Build history of the part. All positions in model axes, mm. Face numbers are marked on the shaded views. Give positions to 0.01 mm unless a question says otherwise; leave off trailing zeros. Loops run counter-clockwise (first coordinate to the right, second up) from the corner with the lowest first, then second, coordinate; pieces in that order, holes last. Notation, with made-up numbers: M -39.5,-8.75 L -34.5,-8.75 A21 cw -34.5,10.25 Z; hole C 51,54 d4. An arc over 180 degrees is marked long. Answer in a Markdown table with one row per item. Add a question column.
```python
from build123d import *

# Parameters (mm, degrees)
BOSS_EXTRUDE1_DEPTH     = 2.5
CUT_EXTRUDE1_DEPTH      = 31.618621785
CUT_EXTRUDE1_DEPTH_BACK = 31.618621785
SKETCH3_W               = 44
SKETCH3_H               = 29
SKETCH3_R               = 1.125
CUT_EXTRUDE2_DEPTH      = 1
BOSS_EXTRUDE2_START     = 0.5
SKETCH3_5_R             = 1.125
BOSS_EXTRUDE2_DEPTH     = 0.5


with BuildPart() as part:
    # Sketch1 → Boss-Extrude1 (new body)
    with BuildSketch(Plane(origin=(0, 0, 0), x_dir=(1, 0, 0), z_dir=(0, 1, 0))):
        with BuildLine():
            Line((22, 17.5), (-22, 17.5))
            ThreePointArc((-22, 17.5), (-24.121320344, 16.621320344), (-25, 14.5))
            Line((-25, 14.5), (-25, 7.5))
            ThreePointArc((-25, 7.5), (-24.12566565, 0), (-25, -7.5))
            Line((-25, -7.5), (-25, -14.5))
            ThreePointArc((-25, -14.5), (-24.121320344, -16.621320344), (-22, -17.5))
            Line((-22, -17.5), (22, -17.5))
            ThreePointArc((22, -17.5), (24.121320344, -16.621320344), (25, -14.5))
            Line((25, -14.5), (25, -7.5))
            ThreePointArc((25, -7.5), (24.12566565, 0), (25, 7.5))
            Line((25, 7.5), (25, 14.5))
            ThreePointArc((25, 14.5), (24.121320344, 16.621320344), (22, 17.5))
        make_face()
    extrude(amount=-BOSS_EXTRUDE1_DEPTH)

    # Sketch2 → Cut-Extrude1 (cut, two sides: drawn at the far end of the back side and taken through both)
    with BuildSketch(Plane.XY.offset(-CUT_EXTRUDE1_DEPTH_BACK)):
        with BuildLine():
            Line((-25, -2.5), (25, -2.5))
            ThreePointArc((25, -2.5), (0, -2.25), (-25, -2.5))
        make_face()
    extrude(amount=CUT_EXTRUDE1_DEPTH + CUT_EXTRUDE1_DEPTH_BACK, mode=Mode.SUBTRACT)

    # Sketch3 → Cut-Extrude2 (cut)
    with BuildSketch(Plane(origin=(0, 0, 0), x_dir=(1, 0, 0), z_dir=(0, 1, 0))):
        Rectangle(SKETCH3_W, SKETCH3_H)
        with Locations(Location((-18.99479618, 11.49479618, 0), (0, 0, 270))):
            Circle(SKETCH3_R, mode=Mode.SUBTRACT)
        with Locations(Location((18.99479618, 11.49479618, 0), (0, 0, 270))):
            Circle(SKETCH3_R, mode=Mode.SUBTRACT)
        with Locations(Location((18.99479618, -11.49479618, 0), (0, 0, 270))):
            Circle(SKETCH3_R, mode=Mode.SUBTRACT)
        with Locations(Location((-18.99479618, -11.49479618, 0), (0, 0, 270))):
            Circle(SKETCH3_R, mode=Mode.SUBTRACT)
    extrude(amount=-CUT_EXTRUDE2_DEPTH, mode=Mode.SUBTRACT)

    # Sketch3_5 → Boss-Extrude2 (add)
    with BuildSketch(Plane(origin=(0, 0, 0), x_dir=(1, 0, 0), z_dir=(0, 1, 0)).offset(BOSS_EXTRUDE2_START)):
        with Locations(Location((-18.99479618, 11.49479618, 0), (0, 0, 270))):
            Circle(SKETCH3_5_R)
        with Locations(Location((18.99479618, 11.49479618, 0), (0, 0, 270))):
            Circle(SKETCH3_5_R)
        with Locations(Location((18.99479618, -11.49479618, 0), (0, 0, 270))):
            Circle(SKETCH3_5_R)
        with Locations(Location((-18.99479618, -11.49479618, 0), (0, 0, 270))):
            Circle(SKETCH3_5_R)
    extrude(amount=-BOSS_EXTRUDE2_DEPTH)


solid = part.part
```
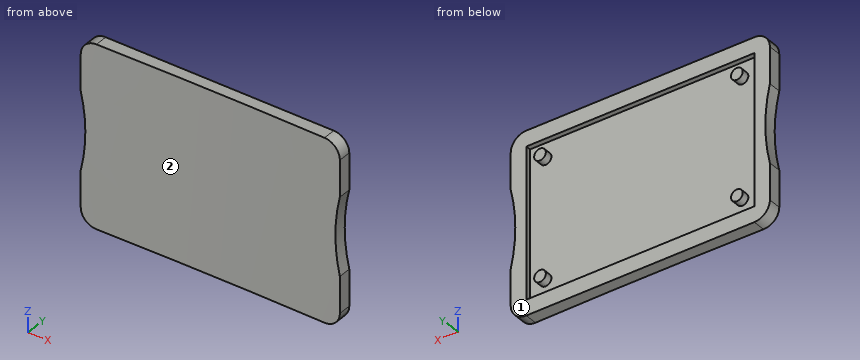
(1) Slice it at C-C, the plane z = -15. Give the cut face in (x, y) (3 decimals), then the cut area to 3 significant figures.
(2) Slice it at A-A, the plane x = -12.5. Give the cut face in (y, z).
(3) Pin check, flat tips, straight feed: pin 1 (0.5 mm diameter, centred on y = -0.5, z = 5, fed in from -X); pin 2 (2 mm diameter, centred on x = 1.5, z = 4, fed in from -Y); pin 3 (0.5 mm diameter, centred on y = -0.5, z = 2.5, fed in from +X). Stop position of each tip, or through.
(4) Wall check: line 1 (Z direction, x = -13, y = -0.5); line 2 (X direction, y = -0.1, z = 0); line 3 (Y direction, x = -2.5, z = 0.5). Give the ranges that are in metal, low to high.
(5) Pull direction X, two halves, no side cores. Call the marked faces 1 and 2: +X half, -X half, draft (parallel to the pull), parting line (faces both ways), or undercut.
(6) Slice it at B-B, the plane z = -8. Give the cut face in (x, y) (3 decimals), then the cut area to 3 significant figures.
Solution:
| question | item | result |
|---|---|---|
| 1 | outline | M -24.958,-2.499 A1250.125 cw 24.958,-2.499 L 24.958,0 L -24.958,0 Z |
| 1 | area | 116 mm^2 |
| 2 | outline | M -2.31,-17.5 L 0,-17.5 L 0,-14.5 L -1,-14.5 L -1,14.5 L 0,14.5 L 0,17.5 L -2.31,17.5 Z |
| 3 | pin 1 | x = -24.55 |
| 3 | pin 2 | y = -2.25 |
| 3 | pin 3 | x = 24.24 |
| 4 | line 1 | -17.5 to -14.5, 14.5 to 17.5 |
| 4 | line 2 | -24.13 to -22, 22 to 24.13 |
| 4 | line 3 | -2.25 to -1 |
| 5 | face 1 | draft |
| 5 | face 2 | undercut |
| 6 | outline | M -25,-2.5 A1250.125 cw 25,-2.5 L 25,0 L 22,0 L 22,-1 L -22,-1 L -22,0 L -25,0 Z |
| 6 | area | 72.7 mm^2 |
